Verification items for the finished model (mm, model axes). A direction names the side the tool comes from. Round coordinates to 2 decimals unless told otherwise and drop trailing zeros. Loops run counter-clockwise (first coordinate to the right, second up) from the corner with the lowest first, then second, coordinate; pieces in that order, holes last. Notation, with made-up numbers: (-27, 39.5) -> (23, 39.5) arc R20 cw to (23, 61.5) -> close; hole circle Ø5 at (-7.5, 64.5). An arc over 180 degrees is marked (long way). Write item = value, one per line. Start each with the question number.
```python
from build123d import *

# Parameters (mm, degrees)
F0_R     = 30
F1_DEPTH = 30
F2_START = 27
F0_R_2   = 2.3
F2_DEPTH = 1
F3_DEPTH = 17
F4_SIZE2 = 16
F4_SIZE  = 25


with BuildPart() as f1:
    # F0 (on Right) → F1 (new body)
    with BuildSketch(Plane.YZ):
        with BuildLine():
            ThreePointArc((45.073977597, -23.8607741614), (49.4963274266, -12.2928260085), (51, 0))
            ThreePointArc((51, 0), (49.4963274266, 12.2928260085), (45.073977597, 23.8607741614))
            ThreePointArc((45.073977597, 23.8607741614), (36.0624458405, 36.0624458405), (23.8607741614, 45.073977597))
            ThreePointArc((23.8607741614, 45.073977597), (0, 51), (-23.8607741614, 45.073977597))
            ThreePointArc((-23.8607741614, 45.073977597), (-36.0624458405, 36.0624458405), (-45.073977597, 23.8607741614))
            ThreePointArc((-45.073977597, 23.8607741614), (-51, 0), (-45.073977597, -23.8607741614))
            ThreePointArc((-45.073977597, -23.8607741614), (-36.0624458405, -36.0624458405), (-23.8607741614, -45.073977597))
            ThreePointArc((-23.8607741614, -45.073977597), (0, -51), (23.8607741614, -45.073977597))
            ThreePointArc((23.8607741614, -45.073977597), (36.0624458405, -36.0624458405), (45.073977597, -23.8607741614))
        make_face()
        Circle(F0_R, mode=Mode.SUBTRACT)
        Circle(F0_R)
    extrude(amount=F1_DEPTH)

    # F0 (on Right) → F2 (join)
    with BuildSketch(Plane.YZ.offset(F2_START)):
        with BuildLine():
            ThreePointArc((23.8607741614, 45.073977597), (36.0624458405, 36.0624458405), (45.073977597, 23.8607741614))
            Line((45.073977597, 23.8607741614), (46.6976567543, 41.2545798264))
            ThreePointArc((46.6976567543, 41.2545798264), (45.2548339959, 45.2548339959), (41.2545798264, 46.6976567543))
            Line((41.2545798264, 46.6976567543), (23.8607741614, 45.073977597))
        make_face()
        with Locations((41.71930009, 41.71930009)):
            Circle(F0_R_2, mode=Mode.SUBTRACT)
        with BuildLine():
            ThreePointArc((-45.073977597, 23.8607741614), (-36.0624458405, 36.0624458405), (-23.8607741614, 45.073977597))
            Line((-23.8607741614, 45.073977597), (-41.2545798264, 46.6976567543))
            ThreePointArc((-41.2545798264, 46.6976567543), (-45.2548339959, 45.2548339959), (-46.6976567543, 41.2545798264))
            Line((-46.6976567543, 41.2545798264), (-45.073977597, 23.8607741614))
        make_face()
        with Locations((-41.71930009, 41.71930009)):
            Circle(F0_R_2, mode=Mode.SUBTRACT)
        with BuildLine():
            Line((-41.2545798264, -46.6976567543), (-23.8607741614, -45.073977597))
            ThreePointArc((-23.8607741614, -45.073977597), (-36.0624458405, -36.0624458405), (-45.073977597, -23.8607741614))
            Line((-45.073977597, -23.8607741614), (-46.6976567543, -41.2545798264))
            ThreePointArc((-46.6976567543, -41.2545798264), (-45.2548339959, -45.2548339959), (-41.2545798264, -46.6976567543))
        make_face()
        with Locations((-41.71930009, -41.71930009)):
            Circle(F0_R_2, mode=Mode.SUBTRACT)
        with BuildLine():
            Line((46.6976567543, -41.2545798264), (45.073977597, -23.8607741614))
            ThreePointArc((45.073977597, -23.8607741614), (36.0624458405, -36.0624458405), (23.8607741614, -45.073977597))
            Line((23.8607741614, -45.073977597), (41.2545798264, -46.6976567543))
            ThreePointArc((41.2545798264, -46.6976567543), (45.2548339959, -45.2548339959), (46.6976567543, -41.2545798264))
        make_face()
        with Locations((41.71930009, -41.71930009)):
            Circle(F0_R_2, mode=Mode.SUBTRACT)
    extrude(amount=F2_DEPTH)

    # F0 (on Right) → F3 (join)
    with BuildSketch(Plane.YZ):
        Circle(F0_R)
    extrude(amount=-F3_DEPTH)

    # F4
    f4_edges = [f1.edges().sort_by_distance(p)[0] for p in [
        (0, -45.073978, 23.860774),
    ]]
    f4_side = f1.faces().sort_by_distance((15, -45.073978, 23.860774))[0]
    chamfer(f4_edges, length=F4_SIZE, length2=F4_SIZE2, reference=f4_side)


solid = f1.part
```
(1) Section check C-C on x = -2.5. Enter the section's corners in (y, z), then the cut area to 3 significant figures.
(2) Section check A-A on y = 0. Enter the section's corners in (x, z).
(3) Access from +Z, -Z, +X, -X, +Y, -Y to the whole of each face (thin tool, end or side, straight path). Record for faces 1 (the flat face through (28, -38, -40)), 2 (the flat face through (28, 38, -38)), 3 (the flat face through (27, 40, 38)), 4 (the flat face through (27, -38, -40)).
(4) Section check B-B on x = 12. Enter the section's corners in (y, z), then the cut area to 3 significant figures.
(5) Scan lines: line 1 (Y direction, x = 18.5, z = -16); line 2 (X direction, y = 45, z = 36); line 3 (Z direction, x = 13, y = -3). Record each from-to range of solid material in increasing order. Write a range as [from, to].
(6) Depth check by flat-ended pin: pin 1 Ø5 at (x, z) = (10.5, 19.5) entering from +Y; pin 2 Ø25 at (y, z) = (38, 38.5) entering from -X; pin 3 Ø11.5 at (y, z) = (-33.5, 32.5) entering from -X; pin 4 Ø25 at (y, z) = (-39.5, -37.5) entering from +X. Enter the tip coordinate at first touch or a pass-through.
(7) Draft check along Y on faces 5 (the cylindrical face through (-8.38, -29.97, 1.32)), 6 (the flat face through (27, -38, 38)), 7 (the cylindrical face through (27.49, -42.02, -39.44)), 8 (the cylindrical face through (27.49, -42.02, 44)). Enter one of: +Y half, -Y half, draft (parallel to the pull), parting line (faces both ways), or undercut.
Computed values:
q1.outline = circle Ø60 at (0, 0)
q1.area = 2,830 mm²
q2.outline = (-17, -30) -> (0, -30) -> (0, -35) -> (25, -51) -> (30, -51) -> (30, 51) -> (25, 51) -> (0, 35) -> (0, 30) -> (-17, 30) -> close
q3.face_1 = -Z, +X, -Y
q3.face_2 = -Z, +X, +Y
q3.face_3 = +Z, -X, +Y
q3.face_4 = -Z, -X, -Y
q4.outline = circle Ø85.36 at (0, 0)
q4.area = 5,720 mm²
q5.line_1 = [-44.02, 44.02]
q5.line_2 = [27, 28]
q5.line_3 = [-43.22, 43.22]
q6.pin_1 = 39.06
q6.pin_2 = 10.3
q6.pin_3 = 9.26
q6.pin_4 = 30
q7.face_5 = parting line
q7.face_6 = draft
q7.face_7 = undercut
q7.face_8 = undercut
